Part model, mm, in its own coordinate system. A direction names the side the tool comes from. Coordinates: 2 decimals unless noted, no trailing zeros. Write each loop counter-clockwise with the first axis right and the second up, starting at its lowest first coordinate (ties: lowest second). Pieces come first, ordered by that corner, then holes. Notation, with made-up numbers: M -12.75,-14.75 L 5.25,-14.75 A19 ccw 5.25,21.25 Z; hole C 64.5,-32.5 d6. An arc over 180 degrees is marked long. Use a Markdown table: item, result. Add a question column.
Q1. Tool access for faces 5 (the flat face through (-1.5, 15, 0)), 6 (the flat face through (-1.25, 11.4, 2.4)), 7 (the flat face through (2.4, 11.4, 1.25)), 8 (the flat face through (-2, 9, 0)): list every direction of +Z, -Z, +X, -X, +Y, -Y with a clear straight run to the whole face (end or side of a thin tool).
Q2. Mould opens along X. For faces 1 (the flat face through (-1.25, 11.4, -2.4)), 2 (the cylindrical face through (-0.45, 6.97, -1.43)), 3 (the flat face through (1.5, 15, 0)), 4 (the flat face through (2.4, 11.4, -1.25)) say: released by +X, released by -X, zero draft, split by the parting line, or undercut.
Q3. Pin check, flat tips, straight feed: pin 1 Ø1.5 at (y, z) = (8, -2.5) entering from -X; pin 2 Ø1.2 at (x, y) = (-2, 10.5) entering from -Z; pin 3 Ø1.5 at (x, z) = (0.5, 0) entering from +Y. Stop position of each tip, or through.
Q4. Slice it at B-B on y = -5.5. Write the cut outline in (x, z), then the cut area to 3 significant figures.
Q5. Wall check: L1, parallel to Z at x = -0.75, y = 14; L2, parallel to X at y = 9.5, z = -0.75. Give the ranges that are in metal, low to high. Write a range as from..to.
Q6. Slice it at A-A on y = 16. Write the cut outline in (x, z).
from build123d import *

# Parameters (mm, degrees)
SKETCH_1_R               = 2.5
EXTRUDE_1_DEPTH          = 8.1
SKETCH_4_R               = 3.5
EXTRUDE_2_DEPTH          = 1
EXTRUDE_3_DEPTH          = 11.4
SKETCH_6_W               = 2.5
SKETCH_6_H               = 1.5
EXTRUDE_4_DEPTH          = 5
CUT_EXTRUDE_2_DEPTH      = 2.5
CUT_EXTRUDE_3_DEPTH      = 2.5
PATTERN_CIRCULAR_4_COUNT = 4
EXTRUDE_6_DEPTH          = 3.6
SKETCH_15_R              = 1.5
EXTRUDE_7_DEPTH          = 3.8
FILLET_2_R               = 1
FILLET_3_R               = 1.75


with BuildPart() as part:
    # Эскиз1 → Бобышка-Вытянуть1 (new body)
    with BuildSketch(Plane(origin=(0, 0, 0), x_dir=(1, 0, 0), z_dir=(0, 1, 0))):
        with Locations(Location((0, 0, 0), (0, 0, 270))):
            Circle(SKETCH_1_R)
    extrude(amount=-EXTRUDE_1_DEPTH)

    # По сечениям1: read off the stored shape, not the designer's step
    # По сечениям1: loft between two sections, ruled curve by curve
    loft_1_from = [
        Edge.make_bspline([(0, 0.5, 3.5), (-7, 0.5, 3.5), (-7, 0.5, -3.5), (0, 0.5, -3.5), (7, 0.5, -3.5), (7, 0.5, 3.5), (0, 0.5, 3.5)], [0, 0, 0, 0, 0.5, 0.5, 0.5, 1, 1, 1, 1], 3, [1, 0.333333333, 0.333333333, 1, 0.333333333, 0.333333333, 1]),
    ]
    loft_1_to = [
        Edge.make_bspline([(-1.133576436, 0, 2.228228997), (-5.59003443, 0, -0.038923874), (-3.322881559, 0, -4.495381869), (1.133576436, 0, -2.228228997), (5.59003443, 0, 0.038923874), (3.322881559, 0, 4.495381869), (-1.133576436, 0, 2.228228997)], [0, 0, 0, 0, 0.5, 0.5, 0.5, 1, 1, 1, 1], 3, [1, 0.333333333, 0.333333333, 1, 0.333333333, 0.333333333, 1]),
    ]
    loft_1 = Solid(Shell([*[Face.make_surface_from_curves(loft_1_from[k], loft_1_to[k]) for k in range(1)], Face(Wire(loft_1_from)), Face(Wire(loft_1_to))]))
    add(loft_1)

    # Эскиз4 → Бобышка-Вытянуть2 (add)
    with BuildSketch(Plane(origin=(0, 0.5, 0), x_dir=(1, 0, 0), z_dir=(0, 1, 0))):
        with Locations(Location((0, 0, 0), (0, 0, 270))):
            Circle(SKETCH_4_R)
    extrude(amount=EXTRUDE_2_DEPTH)

    # Эскиз5 → Бобышка-Вытянуть3 (add)
    with BuildSketch(Plane(origin=(0, 1.5, 0), x_dir=(1, 0, 0), z_dir=(0, 1, 0))):
        Polygon((1.25, 2.5), (1.25, 2), (-1.25, 2), (-1.25, 2.5), (-1.25, 3), (1.25, 3), align=None)
    extrude_3 = extrude(amount=EXTRUDE_3_DEPTH)

    # Эскиз6 → Бобышка-Вытянуть4 (add)
    with BuildSketch(Plane(origin=(0, 12.9, 0), x_dir=(1, 0, 0), z_dir=(0, 1, 0))):
        with Locations((0, 2.25)):
            Rectangle(SKETCH_6_W, SKETCH_6_H)
    extrude_4 = extrude(amount=EXTRUDE_4_DEPTH)

    # Эскиз8 → Вырез-Вытянуть2 (cut)
    with BuildSketch(Plane(origin=(1.25, 0, 0), x_dir=(0, 0, -1), z_dir=(1, 0, 0))):
        Polygon((1.5, 12.9), (2, 12.9), (1.5, 13.4), align=None)
    cut_extrude_2 = extrude(amount=-CUT_EXTRUDE_2_DEPTH, mode=Mode.SUBTRACT)

    # Эскиз9 → Вырез-Вытянуть3 (cut)
    with BuildSketch(Plane(origin=(1.25, 0, 0), x_dir=(0, 0, -1), z_dir=(1, 0, 0))):
        Polygon((1.5, 17.9), (1.5, 17.4), (2, 17.9), align=None)
    cut_extrude_3 = extrude(amount=-CUT_EXTRUDE_3_DEPTH, mode=Mode.SUBTRACT)

    # Круговой массив4: Бобышка-Вытянуть3, Бобышка-Вытянуть4, Вырез-Вытянуть2, Вырез-Вытянуть3 ×4 about axis
    pattern_circular_4_axis = Axis((0, 0, 0), (0, 1, 0))
    add([extrude_3.rotate(pattern_circular_4_axis, i * 360 / PATTERN_CIRCULAR_4_COUNT) for i in range(1, PATTERN_CIRCULAR_4_COUNT)])
    add([extrude_4.rotate(pattern_circular_4_axis, i * 360 / PATTERN_CIRCULAR_4_COUNT) for i in range(1, PATTERN_CIRCULAR_4_COUNT)])
    add([cut_extrude_2.rotate(pattern_circular_4_axis, i * 360 / PATTERN_CIRCULAR_4_COUNT) for i in range(1, PATTERN_CIRCULAR_4_COUNT)], mode=Mode.SUBTRACT)
    add([cut_extrude_3.rotate(pattern_circular_4_axis, i * 360 / PATTERN_CIRCULAR_4_COUNT) for i in range(1, PATTERN_CIRCULAR_4_COUNT)], mode=Mode.SUBTRACT)

    # Эскиз14 → Бобышка-Вытянуть6 (add)
    with BuildSketch(Plane(origin=(0, 1.5, 0), x_dir=(1, 0, 0), z_dir=(0, 1, 0))):
        Polygon((0, 3), (3, 3), (3, -3), (-3, -3), (-3, 3), align=None)
    extrude(amount=EXTRUDE_6_DEPTH)

    # Эскиз15 → Бобышка-Вытянуть7 (add)
    with BuildSketch(Plane(origin=(0, 5.1, 0), x_dir=(1, 0, 0), z_dir=(0, 1, 0))):
        with Locations(Location((0, 0, 0), (0, 0, 90))):
            Circle(SKETCH_15_R)
    extrude(amount=EXTRUDE_7_DEPTH)

    # Скругление2
    fillet_2_edges = [part.edges().sort_by_distance(p)[0] for p in [
        (0, -8.1, -2.5),
    ]]
    fillet(fillet_2_edges, radius=FILLET_2_R)

    # Скругление3
    # the kernel refuses this fillet: 1.75 mm, written as the material it takes off along each edge
    with BuildSketch(Plane(origin=(-3, 1.5, -3), x_dir=(0, 0, 1), z_dir=(0, 1, 0)), Plane(origin=(3, 1.5, -3), x_dir=(-1, 0, 0), z_dir=(0, 1, 0)), Plane(origin=(-3, 1.5, 3), x_dir=(1, 0, 0), z_dir=(0, 1, 0))) as fillet_3_piece_1:
        with BuildLine():
            CenterArc((FILLET_3_R, FILLET_3_R), FILLET_3_R, 180, 90)
            Line((0, FILLET_3_R), (0, 0))
            Line((0, 0), (FILLET_3_R, 0))
        make_face()
    extrude(amount=7.975, mode=Mode.SUBTRACT)
    with BuildSketch(Plane(origin=(3, 1.5, 3), x_dir=(-1, 0, 0), z_dir=(0, 1, 0))) as fillet_3_piece_2:
        with BuildLine():
            CenterArc((FILLET_3_R, -FILLET_3_R), FILLET_3_R, 90, 90)
            Line((0, -FILLET_3_R), (0, 0))
            Line((0, 0), (FILLET_3_R, 0))
        make_face()
    extrude(amount=7.975, mode=Mode.SUBTRACT)


solid = part.part
Recorded:
| question | item | result |
|---|---|---|
| 1 | face 5 | +Z, -Z, +Y |
| 1 | face 6 | +Z, -X, +Y |
| 1 | face 7 | +Z, +X, +Y |
| 1 | face 8 | +Z, -Z |
| 2 | face 1 | released by -X |
| 2 | face 2 | undercut |
| 2 | face 3 | undercut |
| 2 | face 4 | zero draft |
| 3 | pin 1 | x = -1.25 |
| 3 | pin 2 | z = -1.25 |
| 3 | pin 3 | y = 8.9 |
| 4 | outline | C 0,0 d5 |
| 4 | area | 19.6 mm² |
| 5 | L1 | -3..-1.5, 1.5..3 |
| 5 | L2 | -3..-2, 2..3 |
| 6 | outline | M -3,-1.25 L -1.5,-1.25 L -1.5,1.25 L -3,1.25 Z; M -1.25,-3 L 1.25,-3 L 1.25,-1.5 L -1.25,-1.5 Z; M -1.25,1.5 L 1.25,1.5 L 1.25,3 L -1.25,3 Z; M 1.5,-1.25 L 3,-1.25 L 3,1.25 L 1.5,1.25 Z |
